Source: CAD feature listing. Evaluate the final solid. Frame: model axes, mm. A direction names the side the tool comes from. Give positions to 0.01 mm unless a question says otherwise; leave off trailing zeros. Order: outer loops, then holes, each group sorted by start corner. A loop starts at its lowest first (then second) coordinate and runs counter-clockwise, first axis right, second up.
```python
from build123d import *

# Parameters (mm, degrees)
F1_DEPTH = 25.4
F3_DEPTH = 19.05
F4_DEPTH = 19.05
F5_R     = 5.08


with BuildPart() as f1:
    # F0 (on Front) → F1 (new body)
    with BuildSketch(Plane.XZ):
        with BuildLine():
            ThreePointArc((35.395226, 0), (25.519415, 37.09865), (0, 65.779671))
            ThreePointArc((0, 65.779671), (-27.871905, 38.118795), (-37.301891, 0))
            Line((-37.301891, 0), (-22.862449, -70.993923))
            Line((-22.862449, -70.993923), (19.653682, -70.993923))
            Line((19.653682, -70.993923), (35.395226, 0))
        make_face()
    extrude(amount=F1_DEPTH)

    # F2 (on face) → F3 (cut)
    with BuildSketch(Plane(origin=(0, 0, 0), x_dir=(-1, 0, 0), z_dir=(0, 1, 0))):
        with BuildLine():
            ThreePointArc((26.61556, 0), (22.594878, 30.780864), (0, 52.066986))
            ThreePointArc((0, 52.066986), (-16.922181, 28.453793), (-22.78091, 0))
            Line((-22.78091, 0), (-9.381168, -60.432459))
            Line((-9.381168, -60.432459), (13.559343, -60.432459))
            Line((13.559343, -60.432459), (26.61556, 0))
        make_face()
    extrude(amount=F3_DEPTH, mode=Mode.SUBTRACT)

    # F2 (on face) → F4 (cut)
    with BuildSketch(Plane(origin=(0, 0, 0), x_dir=(-1, 0, 0), z_dir=(0, 1, 0))):
        with BuildLine():
            ThreePointArc((26.61556, 0), (22.594878, 30.780864), (0, 52.066986))
            ThreePointArc((0, 52.066986), (-16.922181, 28.453793), (-22.78091, 0))
            Line((-22.78091, 0), (-9.381168, -60.432459))
            Line((-9.381168, -60.432459), (13.559343, -60.432459))
            Line((13.559343, -60.432459), (26.61556, 0))
        make_face()
    extrude(amount=-F4_DEPTH, mode=Mode.SUBTRACT)

    # F5
    f5_edges = [f1.edges().sort_by_distance(p)[0] for p in [
        (27.524454, 0, -35.496961),
        (27.524454, -25.4, -35.496961),
        (19.653682, -12.7, -70.993923),
        (-1.604384, 0, -70.993923),
        (-1.604384, -25.4, -70.993923),
        (-22.862449, -12.7, -70.993923),
        (-30.08217, 0, -35.496961),
        (-30.08217, -25.4, -35.496961),
    ]]
    fillet(f5_edges, radius=F5_R)


solid = f1.part
```
1) Section query D-D, the plane y = -23.5. Return the cut outline in (x, z), and give its area (3 significant figures).
Report:
outline: (-37.27, 5.44) - (-22.59, -66.7) arc R3.96 ccw to (-18.71, -69.88) - (15.58, -69.88) arc R3.96 ccw to (19.44, -66.77) - (35.18, 4.19) arc R82.97 ccw to (0, 65.78) arc R72.73 ccw to start
area: 7,250 mm2
2) Section query C-C, the plane z = 24. Return the cut outline in (x, y).
Report:
outline: (-34.01, -25.4) - (31.17, -25.4) - (31.17, 0) - (18.69, 0) - (18.69, -19.05) - (-25.41, -19.05) - (-25.41, 0) - (-34.01, 0) - close
3) Reachability of faces 1 (the flat face through (16.175, -9.392, -29.793)), 2 (the cylindrical face through (28.244, -1.528, -25.558)) from +Z, -Z, +X, -X, +Y, -Y: full face, straight path, thin tool, end or side. Return the list, or none.
Report:
face 1: +Y
face 2: -Z, +X, +Y
4) Section query A-A, the plane y = -9. Return the cut outline in (x, z).
Report:
outline: (-37.3, 0) - (-23.69, -66.93) arc R5.08 ccw to (-18.71, -70.99) - (15.58, -70.99) arc R5.08 ccw to (20.54, -67.01) - (35.4, 0) arc R82.97 ccw to (0, 65.78) arc R72.73 ccw to start; hole (-26.62, 0) - (-13.56, -60.43) - (9.38, -60.43) - (22.78, 0) arc R69.89 ccw to (0, 52.07) arc R46.19 ccw to start
5) Pin query (flat end, axial travel): pin 1 (15 mm diameter, centred on x = -2.5, y = -12, fed in from +Z); pin 2 (12 mm diameter, centred on y = -8, z = -55, fed in from -X); pin 3 (15 mm diameter, centred on x = -12.5, z = -1.5, fed in from +Y). Return the tip coordinate at first contact, or that it passes through.
Report:
pin 1: stops at z = 65.78
pin 2: stops at x = -27.34
pin 3: stops at y = -19.05
6) Section query B-B, the plane x = 5. Return the cut outline in (y, z), and give its area (3 significant figures).
Report:
outline: (-25.4, -65.91) arc R5.08 ccw to (-20.32, -70.99) - (-5.08, -70.99) arc R5.08 ccw to (0, -65.91) - (0, -60.43) - (-19.05, -60.43) - (-19.05, 47.02) - (0, 47.02) - (0, 61.99) - (-25.4, 61.99) - close
area: 1,320 mm2
7) Draft query along Z for faces 3 (the cylindrical face through (-22.795, -9.392, 30.385)), 4 (the flat face through (-30.591, -12.593, -32.995)), 5 (the flat face through (-2, -25.4, 1)). Return one class per face: +Z half, -Z half, draft (parallel to the pull), parting line (faces both ways), or undercut.
Report:
face 3: undercut
face 4: -Z half
face 5: draft
8) Material intervals for L1, parallel to X at y = -13.25, z = 9.5; L2, parallel to Y at x = 8.5, z = -57.5; L3, parallel to X at y = -11.5, z = 47.5, sorted ascending.
Report:
L1: x = -36.97 to -27.66, 22.19 to 34.59
L2: y = -25.4 to -19.05
L3: x = -21.54 to -8.09, 4.56 to 18.88
